Can you work these out from the model? Positions are in its coordinate system, mm. Coordinates: 2 decimals unless noted, no trailing zeros. Order: outer loops, then holes, each group sorted by start corner. A loop starts at its lowest first (then second) coordinate and runs counter-clockwise, first axis right, second up. Notation, with made-up numbers: (-32, -30.5) -> (22, -30.5) arc R18 ccw to (22, -3.5) -> close; hole circle Ø9 at (-8.75, 38.5). An arc over 180 degrees is marked (long way). Answer in a Markdown table with one row per item. Add a question column.
1. Imagine slicing it at B-B on y = 46. Write out the boundary of the cut face in (x, z).
2. Imagine slicing it at A-A on x = -38. Write out the boundary of the cut face in (y, z), plus the area to 3 significant figures.
3. If I drill on line 1 along Y through (x, z) = (-38, -0.15); line 2 along X through (y, z) = (46, 0.45), over which ranges is the centre line in solid material (lowest first)? Write a range as [from, to].
4. We'd pull the mould along Y, two halves only. Please class faces 1 (the face through (1, -1, 0.794)), 2 (the face through (-37.2, -47.5, 0)): pulls with the +Y half, pulls with the -Y half, needs draft (parallel to the pull), parting line crosses it, or undercut.
from build123d import *

# Parameters (mm, degrees)
SKETCH1_W           = 1.5875
SKETCH1_H           = 99.999999898
BOSS_EXTRUDE1_DEPTH = 41.999999947
SKETCH2_R           = 1.700000029
CUT_EXTRUDE1_DEPTH  = 66.318604905


with BuildPart() as part:
    # Sketch1 → Boss-Extrude1 (new, symmetric)
    with BuildSketch(Plane(origin=(0, 0, 0), x_dir=(0, 0, -1), z_dir=(1, 0, 0))):
        Rectangle(SKETCH1_W, SKETCH1_H)
    extrude(amount=BOSS_EXTRUDE1_DEPTH, both=True)

    # Sketch2 → Cut-Extrude1 (cut, through all)
    with BuildSketch(Plane.XY.offset(0.79375)):
        with Locations((-37.999999819, 45.999999821)):
            Circle(SKETCH2_R)
        with Locations((37.999999819, 45.999999821)):
            Circle(SKETCH2_R)
        with Locations((37.999999819, -45.999999821)):
            Circle(SKETCH2_R)
        with Locations((-37.999999819, -45.999999821)):
            Circle(SKETCH2_R)
    extrude(amount=-CUT_EXTRUDE1_DEPTH, mode=Mode.SUBTRACT)


solid = part.part
Answers follow:
| question | item | result |
|---|---|---|
| 1 | outline | (-42, -0.79) -> (-39.7, -0.79) -> (-39.7, 0.79) -> (-42, 0.79) -> close; (-36.3, -0.79) -> (36.3, -0.79) -> (36.3, 0.79) -> (-36.3, 0.79) -> close; (39.7, -0.79) -> (42, -0.79) -> (42, 0.79) -> (39.7, 0.79) -> close |
| 2 | outline | (-50, -0.79) -> (-47.7, -0.79) -> (-47.7, 0.79) -> (-50, 0.79) -> close; (-44.3, -0.79) -> (44.3, -0.79) -> (44.3, 0.79) -> (-44.3, 0.79) -> close; (47.7, -0.79) -> (50, -0.79) -> (50, 0.79) -> (47.7, 0.79) -> close |
| 2 | area | 148 mm² |
| 3 | line 1 | y = [-50, -47.7], [-44.3, 44.3], [47.7, 50] |
| 3 | line 2 | x = [-42, -39.7], [-36.3, 36.3], [39.7, 42] |
| 4 | face 1 | needs draft |
| 4 | face 2 | undercut |
